Geometry check sheet. Reference: the model listing, model coordinates, mm. Face numbers are marked on the shaded views. A direction names the side the tool comes from. Coordinates: 2 decimals unless noted, no trailing zeros. Loops run counter-clockwise (first coordinate to the right, second up) from the corner with the lowest first, then second, coordinate; pieces in that order, holes last. Notation, with made-up numbers: (40, -20) -> (90, -20) arc R15 ccw to (90, 3) -> close; hole circle Ø10 at (16.25, 22). An arc over 180 degrees is marked (long way). Answer as a JSON object with one key per item and string values.
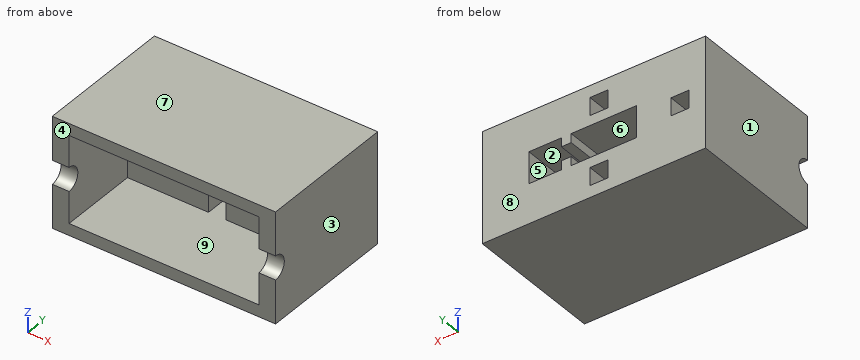
from build123d import *

# Parameters (mm, degrees)
SKETCH1_W                = 143.51
SKETCH1_H                = 121.92
BIG_BLOCK_DEPTH          = 88.9
SERVO_CUTOUT_DEPTH       = 25.654
SKETCH3_W                = 121.92
SKETCH3_H                = 55.88
CUT_EXTRUDE2_DEPTH       = 50.8
CUT_EXTRUDE18_DEPTH      = 172.184986353
CUT_EXTRUDE18_DEPTH_BACK = 48.26
SKETCH6_W                = 20.822928363
SKETCH6_H                = 20.278092026
SKETCH10_W               = 11.43
SKETCH10_H               = 11.43
CUT_EXTRUDE19_DEPTH      = 187.082964166
SKETCH11_W               = 11.43
SKETCH11_H               = 11.43
CUT_EXTRUDE20_DEPTH      = 187.082964166
SKETCH9_W                = 11.43
SKETCH9_H                = 11.43
CUT_EXTRUDE22_DEPTH      = 187.082964166
SKETCH12_W               = 143.51
SKETCH12_H               = 25.4
REMOVESIDES_DEPTH        = 187.082964166
CUT_EXTRUDE23_DEPTH      = 189.901333259
CUT_EXTRUDE23_DEPTH_BACK = 189.901333259


with BuildPart() as part:
    # Sketch1 → Big Block (new body)
    with BuildSketch(Plane(origin=(0, 0, 0), x_dir=(1, 0, 0), z_dir=(0, 1, 0))):
        with Locations((-49.021531365, -49.206642066)):
            Rectangle(SKETCH1_W, SKETCH1_H)
    extrude(amount=BIG_BLOCK_DEPTH)

    # Sketch2 → Servo Cutout (cut)
    with BuildSketch(Plane(origin=(0, 88.9, 0), x_dir=(1, 0, 0), z_dir=(0, 1, 0))):
        Polygon((-76.326531365, -39.046642066), (-34.416531365, -39.046642066), (-34.416531365, -44.761642066), (-19.176531365, -44.761642066), (-19.176531365, -53.651642066), (-34.416531365, -53.651642066), (-34.416531365, -59.366642066), (-76.326531365, -59.366642066), align=None)
    extrude(amount=-SERVO_CUTOUT_DEPTH, mode=Mode.SUBTRACT)

    # Sketch3 → Cut-Extrude2 (cut)
    with BuildSketch(Plane(origin=(0, 0, 0), x_dir=(-1, 0, 0), z_dir=(0, -1, 0))):
        with Locations((49.021531365, -49.206642066)):
            Rectangle(SKETCH3_W, SKETCH3_H)
    extrude(amount=-CUT_EXTRUDE2_DEPTH, mode=Mode.SUBTRACT)

    # Sketch6 → Cut-Extrude18 (cut, two sides: drawn at the far end of the back side and taken through both)
    with BuildSketch(Plane.XZ.offset(-50.8).offset(-CUT_EXTRUDE18_DEPTH_BACK)):
        with Locations((-17.655067184, 49.185688079)):
            Rectangle(SKETCH6_W, SKETCH6_H)
    extrude(amount=CUT_EXTRUDE18_DEPTH + CUT_EXTRUDE18_DEPTH_BACK, mode=Mode.SUBTRACT)

    # Sketch10 → Cut-Extrude19 (cut, through all)
    with BuildSketch(Plane(origin=(0, 88.9, 0), x_dir=(1, 0, 0), z_dir=(0, 1, 0))):
        with Locations((-52.196531365, -26.981642066)):
            Rectangle(SKETCH10_W, SKETCH10_H)
    extrude(amount=-CUT_EXTRUDE19_DEPTH, mode=Mode.SUBTRACT)

    # Sketch11 → Cut-Extrude20 (cut, through all)
    with BuildSketch(Plane(origin=(0, 88.9, 0), x_dir=(1, 0, 0), z_dir=(0, 1, 0))):
        with Locations((-52.196531365, -71.431642066)):
            Rectangle(SKETCH11_W, SKETCH11_H)
    extrude(amount=-CUT_EXTRUDE20_DEPTH, mode=Mode.SUBTRACT)

    # Sketch9 → Cut-Extrude22 (cut, through all)
    with BuildSketch(Plane(origin=(0, 88.9, 0), x_dir=(1, 0, 0), z_dir=(0, 1, 0))):
        with Locations((-104.266531365, -49.206642066)):
            Rectangle(SKETCH9_W, SKETCH9_H)
    extrude(amount=-CUT_EXTRUDE22_DEPTH, mode=Mode.SUBTRACT)

    # Sketch12 → removesides (cut, through all)
    with BuildSketch(Plane(origin=(0, 0, 0), x_dir=(-1, 0, 0), z_dir=(0, -1, 0))):
        with Locations((49.021531365, -97.466642066)):
            Rectangle(SKETCH12_W, SKETCH12_H)
        with Locations((49.021531365, -0.946642066)):
            Rectangle(SKETCH12_W, SKETCH12_H)
    extrude(amount=-REMOVESIDES_DEPTH, mode=Mode.SUBTRACT)

    # Sketch13 → Cut-Extrude23 (cut, two sides: drawn at the far end of the back side and taken through both)
    with BuildSketch(Plane.ZY.offset(120.776531365).offset(-CUT_EXTRUDE23_DEPTH_BACK)):
        with BuildLine():
            Line((41.586642066, 0), (56.826642066, 0))
            ThreePointArc((56.826642066, 0), (49.206642066, 7.62), (41.586642066, 0))
        make_face()
    extrude(amount=CUT_EXTRUDE23_DEPTH + CUT_EXTRUDE23_DEPTH_BACK, mode=Mode.SUBTRACT)


solid = part.part
1. Tool access check on the marked faces 5, 6, 7, 8 and 9. Record the directions out of +Z, -Z, +X, -X, +Y, -Y that give a thin tool (end or side, any length) a straight path to the whole face; none if there is none.
Evaluation:
{"face 5": "+Y, -Y", "face 6": "+Y", "face 7": "+Z, +X, -X, +Y, -Y", "face 8": "+Z, -Z, +X, -X, +Y", "face 9": "-Y"}
2. Depth check by flat-ended pin: P1, Ø12, axis at x = -14.5, z = 30, coming from the -Y side. Enter the tip coordinate at first touch or a pass-through.
Evaluation:
{"P1": "stops at y = 50.8"}
3. Mould release check, pull along X, two halves, no side actions. Record for the marked faces 1, 2, 3 and 4: released by +X, released by -X, zero draft, split by the parting line, or undercut.
Evaluation:
{"face 1": "released by -X", "face 2": "undercut", "face 3": "released by +X", "face 4": "zero draft"}
4. Section check D-D, the plane x = -15. Record the boundary of the cut face in (y, z), then the cut area to 3 significant figures.
Evaluation:
{"outline": "(0, 13.65) -> (88.9, 13.65) -> (88.9, 39.05) -> (50.8, 39.05) -> (50.8, 21.27) -> (0, 21.27) -> close; (0, 77.15) -> (50.8, 77.15) -> (50.8, 59.32) -> (88.9, 59.32) -> (88.9, 84.77) -> (0, 84.77) -> close", "area": "2,710 mm^2"}
5. Section check C-C, the plane z = 26.5. Record the boundary of the cut face in (x, y), then the cut area to 3 significant figures.
Evaluation:
{"outline": "(-120.78, 0) -> (-109.98, 0) -> (-109.98, 50.8) -> (-57.91, 50.8) -> (-57.91, 88.9) -> (-120.78, 88.9) -> close; (-46.48, 50.8) -> (11.94, 50.8) -> (11.94, 0) -> (22.73, 0) -> (22.73, 88.9) -> (-46.48, 88.9) -> close", "area": "6,130 mm^2"}
6. Section check B-B, the plane x = -48. Record the boundary of the cut face in (y, z).
Evaluation:
{"outline": "(0, 13.65) -> (88.9, 13.65) -> (88.9, 21.27) -> (0, 21.27) -> close; (0, 77.15) -> (88.9, 77.15) -> (88.9, 84.77) -> (0, 84.77) -> close; (50.8, 32.7) -> (88.9, 32.7) -> (88.9, 39.05) -> (63.25, 39.05) -> (63.25, 59.37) -> (88.9, 59.37) -> (88.9, 65.72) -> (50.8, 65.72) -> close"}
7. Thickness scan on probe 1 along Z at (x, y) = (-48.5, 74); probe 2 along Z at (x, y) = (-49, 25.5); probe 3 along X at (y, z) = (24, 27.5). Record the ranges inside material, lowest first. Write a range as from..to.
Evaluation:
{"probe 1": "z = 13.65..21.27, 32.7..39.05, 59.37..65.72, 77.15..84.77", "probe 2": "z = 13.65..21.27, 77.15..84.77", "probe 3": "x = -120.78..-109.98, 11.94..22.73"}
8. Section check A-A, the plane y = 76.5. Record the boundary of the cut face in (x, z), then the cut area to 3 significant figures.
Evaluation:
{"outline": "(-120.78, 13.65) -> (22.73, 13.65) -> (22.73, 84.77) -> (-120.78, 84.77) -> close; hole (-109.98, 43.49) -> (-98.55, 43.49) -> (-98.55, 54.92) -> (-109.98, 54.92) -> close; hole (-76.33, 39.05) -> (-34.42, 39.05) -> (-34.42, 44.76) -> (-28.07, 44.76) -> (-28.07, 39.05) -> (-7.24, 39.05) -> (-7.24, 59.32) -> (-28.07, 59.32) -> (-28.07, 53.65) -> (-34.42, 53.65) -> (-34.42, 59.37) -> (-76.33, 59.37) -> close; hole (-57.91, 21.27) -> (-46.48, 21.27) -> (-46.48, 32.7) -> (-57.91, 32.7) -> close; hole (-57.91, 65.72) -> (-46.48, 65.72) -> (-46.48, 77.15) -> (-57.91, 77.15) -> close", "area": "8,480 mm^2"}
